Could you check a few things on this drawing? It's one solid part, dimensions in mm from its lowest x, y, z. A direction names the side the tool comes from. Coordinates: 2 decimals unless noted, no trailing zeros. Write each loop counter-clockwise with the first axis right and the second up, starting at its lowest first coordinate (ties: lowest second). Pieces come first, ordered by that corner, then holes. Notation, with made-up numbers: M 45,49 L 95,49 A17 ccw 95,64 Z; hole C 62.25,50.5 d5. An arc over 180 degrees is marked long. Use a Markdown table: item, result.
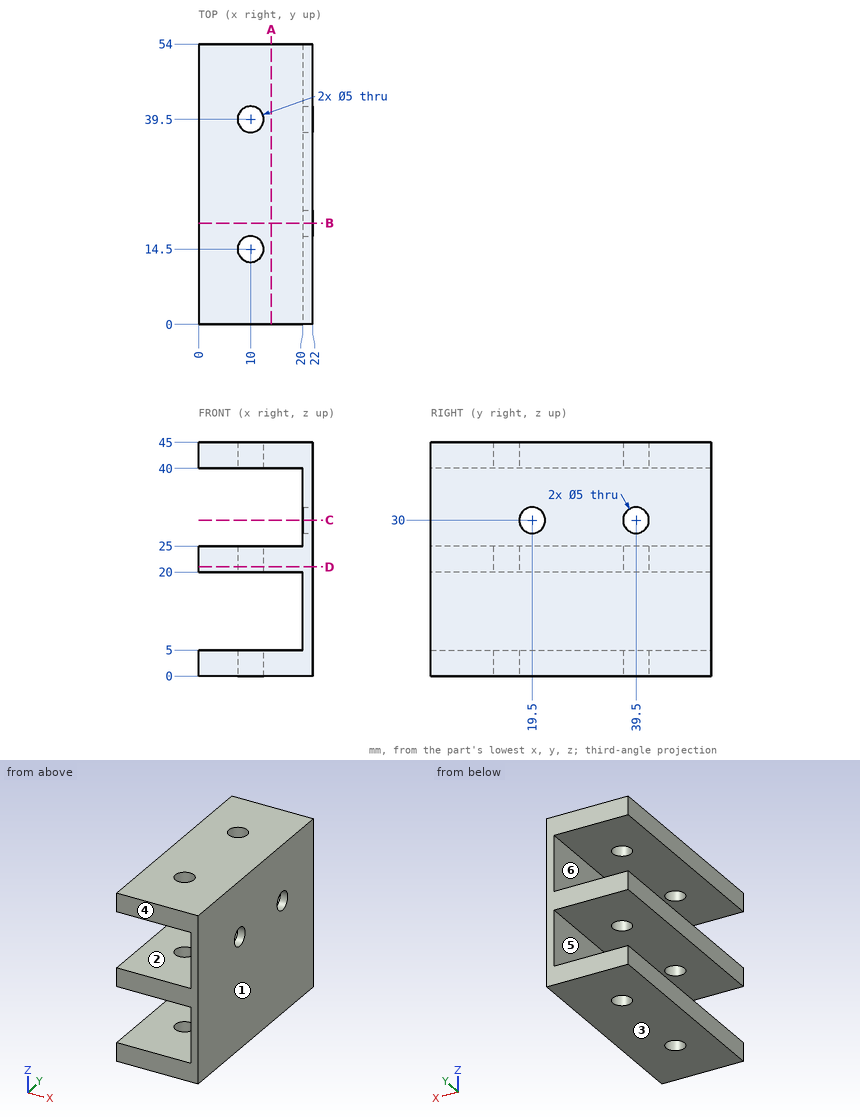
1. Suppose I cut it at D-D on z = 21. Write out the boundary of the cut face in (x, y).
Answers follow:
| item | result |
|---|---|
| outline | M 0,0 L 22,0 L 22,54 L 0,54 Z; hole C 10,14.5 d5; hole C 10,39.5 d5 |
2. I need wall thicknesses on probe 1 along Z at (x, y) = (10.75, 28.5); probe 2 along Z at (x, y) = (21.55, 19.5); probe 3 along Y at (x, z) = (10, 1.7). Which ranges of each line are inside material? Lowest first, please.
Answers follow:
| item | result |
|---|---|
| probe 1 | z = 0 to 5, 20 to 25, 40 to 45 |
| probe 2 | z = 0 to 27.5, 32.5 to 45 |
| probe 3 | y = 0 to 12, 17 to 37, 42 to 54 |
3. Suppose I cut it at B-B on y = 19.5. Write out the boundary of the cut face in (x, z), and give its area (3 significant figures).
Answers follow:
| item | result |
|---|---|
| outline | M 0,0 L 22,0 L 22,27.5 L 20,27.5 L 20,25 L 0,25 L 0,20 L 20,20 L 20,5 L 0,5 Z; M 0,40 L 20,40 L 20,32.5 L 22,32.5 L 22,45 L 0,45 Z |
| area | 380 mm2 |
4. We'd pull the mould along Z, two halves only. Please class the marked faces 3, 4, 5 and 6: +Z half, -Z half, draft (parallel to the pull), parting line (faces both ways), or undercut.
Answers follow:
| item | result |
|---|---|
| face 3 | -Z half |
| face 4 | draft |
| face 5 | undercut |
| face 6 | undercut |
5. Suppose I cut it at C-C on z = 30. Write out the boundary of the cut face in (x, y), and give its area (3 significant figures).
Answers follow:
| item | result |
|---|---|
| outline | M 20,0 L 22,0 L 22,17 L 20,17 Z; M 20,22 L 22,22 L 22,37 L 20,37 Z; M 20,42 L 22,42 L 22,54 L 20,54 Z |
| area | 88.0 mm2 |
6. Which directions (+Z, -Z, +X, -X, +Y, -Y) give clear straight access to the entire face, cutting with the end or side of a thin tool? Please do the marked faces 1 and 2.
Answers follow:
| item | result |
|---|---|
| face 1 | +Z, -Z, +X, +Y, -Y |
| face 2 | -X, +Y, -Y |
7. Suppose I cut it at A-A on x = 14. Write out the boundary of the cut face in (y, z), and give its area (3 significant figures).
Answers follow:
| item | result |
|---|---|
| outline | M 0,0 L 54,0 L 54,5 L 0,5 Z; M 0,20 L 54,20 L 54,25 L 0,25 Z; M 0,40 L 54,40 L 54,45 L 0,45 Z |
| area | 810 mm2 |
8. Will this pin go through, and if not, where does the flat tip stop? pin 1 Ø6.5 at (y, z) = (39.5, 30) entering from -X.
Answers follow:
| item | result |
|---|---|
| pin 1 | stops at x = 20 |
